from build123d import *

# Parameters (mm, degrees)
SKETCH_W        = 56
SKETCH_H        = 88
PAD_DEPTH       = 4
SKETCH004_R     = 1.8
POCKET001_DEPTH = 5


with BuildPart() as part:
    # Sketch → Pad (new body)
    with BuildSketch(Plane.XY):
        Rectangle(SKETCH_W, SKETCH_H)
    extrude(amount=PAD_DEPTH)

    # Sketch004 → Pocket001 (cut)
    with BuildSketch(Plane(origin=(0, 0, 0), x_dir=(1, 0, 0), z_dir=(0, 0, -1))):
        with Locations((0, -35)):
            Circle(SKETCH004_R)
        with Locations((15, -35)):
            Circle(SKETCH004_R)
        with Locations((-15, -35)):
            Circle(SKETCH004_R)
        with Locations((15, 35)):
            Circle(SKETCH004_R)
        with Locations((0, 35)):
            Circle(SKETCH004_R)
        with Locations((-15, 35)):
            Circle(SKETCH004_R)
    extrude(amount=-POCKET001_DEPTH, mode=Mode.SUBTRACT)


solid = part.part
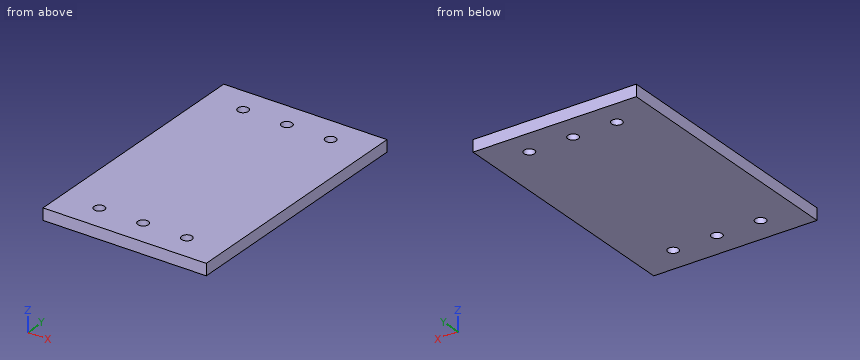
Model file for the job. Use its own axes, mm. Give positions to 0.01 mm unless a question says otherwise; leave off trailing zeros. Write each loop counter-clockwise with the first axis right and the second up, starting at its lowest first coordinate (ties: lowest second). Pieces come first, ordered by that corner, then holes. Notation, with made-up numbers: M -23,55 L 22,55 A32 ccw 22,84 Z; hole C 84,77 d4. An arc over 180 degrees is marked long. One line per item, written item: value. Start each with the question number.
Q1. Probe probe 1 along Y at (x, z) = (15, 2.35); probe 2 along X at (y, z) = (35, 3.7); probe 3 along X at (y, z) = (-34, 0.7). List the from-to ranges inside material, lowest first. Write a range as [from, to].
Q2. Saw through at B-B, the plane x = -15. Write the cut outline in (y, z).
Q3. Drop flat-ended pins along their axis: pin 1 Ø6 at (x, y) = (15, 35) entering from -Z; pin 2 Ø3 at (x, y) = (0, -35) entering from -Z. Give the stop position or say it passes through.
Q4. Saw through at A-A, the plane y = -35. Write the cut outline in (x, z).
Output values:
1. probe 1: y = [-44, -36.8], [-33.2, 33.2], [36.8, 44]
1. probe 2: x = [-28, -16.8], [-13.2, -1.8], [1.8, 13.2], [16.8, 28]
1. probe 3: x = [-28, -16.5], [-13.5, -1.5], [1.5, 13.5], [16.5, 28]
2. outline: M -44,0 L -36.8,0 L -36.8,4 L -44,4 Z; M -33.2,0 L 33.2,0 L 33.2,4 L -33.2,4 Z; M 36.8,0 L 44,0 L 44,4 L 36.8,4 Z
3. pin 1: stops at z = 0
3. pin 2: passes through
4. outline: M -28,0 L -16.8,0 L -16.8,4 L -28,4 Z; M -13.2,0 L -1.8,0 L -1.8,4 L -13.2,4 Z; M 1.8,0 L 13.2,0 L 13.2,4 L 1.8,4 Z; M 16.8,0 L 28,0 L 28,4 L 16.8,4 Z
